Autodesk Inventor part; units mm, degrees
ref_plane "YZ Plane" through (0, 0, 0) normal (1, 0, 0) x (0, 1, 0)
ref_plane "XZ Plane" through (0, 0, 0) normal (0, 1, 0) x (-1, 0, 0)
ref_plane "XY Plane" through (0, 0, 0) normal (0, 0, 1) x (1, 0, 0)
sketch "スケッチ1" plane through (0, 0, 0) normal (0, 1, 0) x (-1, 0, 0)
  line L0 (0, 0) -> (15, 0)
  line L1 (40, 0) -> (40, -7.5) construction
  line L2 (40, -30) -> (15, -30) construction
  line L3 (0, -30) -> (0, 0)
  line L4 (40, -7.5) -> (40, -22.5)
  line L5 (40, -7.5) -> (55, -7.5) construction
  line L6 (40, -22.5) -> (15, -30)
  line L7 (40, -7.5) -> (15, 0)
  line L8 (15, 0) -> (40, 0) construction
  line L9 (40, -7.5) -> (40, -22.5)
  line L10 (40, -22.5) -> (40, -30) construction
  line L11 (15, -30) -> (0, -30)
  dimension "d0" = 40
  dimension "d1" = 30
  dimension "d2" = 7.5
  dimension "d3" = 15
  dimension "d4" = 90
  dimension "d5" = 15
  dimension "d6" = 15
extrude "押し出し1" add sketch "スケッチ1" along normal blind 3
sketch "スケッチ2" plane through (0, 3, 0) normal (0, 1, 0) x (1, 0, 0)
  line L0 (0, 0) -> (0, 30)
  line L1 (-15, 0) -> (0, 0)
  point P0 (-35, 15)
  point P1 (-35, 15)
  point P2 (-25, 15)
  point P3 (-7.5, 15)
  point P4 (-7.5, 5)
  point P5 (-7.5, 25)
  dimension "d9" = 35
  dimension "d10" = 15
  dimension "d11" = 10
  dimension "d12" = 7.5
  dimension "d13" = 15
  dimension "d14" = 10
  dimension "d15" = 10
hole "穴1" at (-35, 3, -15) at (-25, 3, -15) at (-7.5, 3, -15) at (-7.5, 3, -5) at (-7.5, 3, -25) direction (0, -1, 0) diameter 3.2 end through all
fillet "フィレット1" radius 2 6 edges at (-15, 1.5, 0) (0, 1.5, 0) (0, 1.5, -30) (-40, 1.5, -7.5) (-40, 1.5, -22.5) (-15, 1.5, -30)
properties part number "射出_固定5" material "アルミニウム 6061"
Part model, mm, in its own coordinate system. Round coordinates to 2 decimals unless told otherwise and drop trailing zeros. Order: outer loops, then holes, each group sorted by start corner. A loop starts at its lowest first (then second) coordinate and runs counter-clockwise, first axis right, second up. Notation, with made-up numbers: M 21,85.25 L 64,85.25 A23 ccw 64,121.25 Z; hole C 36,7.5 d1. An arc over 180 degrees is marked long. Answer in a Markdown table with one row per item. Add a question column.
Q1. Wall check: L1, parallel to X at y = 0.9, z = -15; L2, parallel to Z at x = -25, y = 1.9; L3, parallel to Z at x = -35, y = 1.1. Give the ranges that are in metal, low to high. Write a range as from..to.
Q2. Cut at B-B on y = 2.5. Give the cut face in (x, z).
Q3. Cut at D-D on z = -25. Give the cut face in (x, y).
Q4. Pin check, flat tips, straight feed: pin 1 (3.5 mm diameter, centred on x = -7.5, z = -5, fed in from -Y); pin 2 (2.5 mm diameter, centred on x = -7.5, z = -25, fed in from +Y); pin 3 (1.5 mm diameter, centred on x = -23, y = 1, fed in from -Z) (3 decimals); pin 4 (1 mm diameter, centred on x = -26, y = 0.5, fed in from +Z). Stop position of each tip, or through.
Q5. Cut at A-A on x = -7.5. Give the cut face in (y, z).
Q6. Mould opens along X. For faces 1 (the face through (-6.53, 1.48, -16.27)), 2 (the face through (-27.091, 1.479, -3.627)), 3 (the face through (-5.94, 1.48, -5.35)), 4 (the face through (-0.57, 1.52, -29.4)) say: +X half, -X half, draft (parallel to the pull), parting line (faces both ways), or undercut.
Q7. Cut at C-C on x = -36. Give the cut face in (y, z), and give its area (3 significant figures).
Established:
| question | item | result |
|---|---|---|
| 1 | L1 | x = -40..-36.6, -33.4..-26.6, -23.4..-9.1, -5.9..0 |
| 1 | L2 | z = -27..-16.6, -13.4..-3 |
| 1 | L3 | z = -24..-16.6, -13.4..-6 |
| 2 | outline | M -40,-21.01 A2 ccw -38.57,-22.93 L -15.28,-29.92 A2 ccw -14.71,-30 L -2,-30 A2 ccw 0,-28 L 0,-2 A2 ccw -2,0 L -14.71,0 A2 ccw -15.28,-0.08 L -38.57,-7.07 A2 ccw -40,-8.99 Z; hole C -35,-15 d3.2; hole C -25,-15 d3.2; hole C -7.5,-25 d3.2; hole C -7.5,-15 d3.2; hole C -7.5,-5 d3.2 |
| 3 | outline | M -31.67,0 L -9.1,0 L -9.1,3 L -31.67,3 Z; M -5.9,0 L 0,0 L 0,3 L -5.9,3 Z |
| 4 | pin 1 | stops at y = 0 |
| 4 | pin 2 | passes through |
| 4 | pin 3 | stops at z = -27.825 |
| 4 | pin 4 | stops at z = -3.15 |
| 5 | outline | M 0,-30 L 3,-30 L 3,-26.6 L 0,-26.6 Z; M 0,-23.4 L 3,-23.4 L 3,-16.6 L 0,-16.6 Z; M 0,-13.4 L 3,-13.4 L 3,-6.6 L 0,-6.6 Z; M 0,-3.4 L 3,-3.4 L 3,0 L 0,0 Z |
| 6 | face 1 | undercut |
| 6 | face 2 | -X half |
| 6 | face 3 | undercut |
| 6 | face 4 | +X half |
| 7 | outline | M 0,-23.7 L 3,-23.7 L 3,-16.25 L 0,-16.25 Z; M 0,-13.75 L 3,-13.75 L 3,-6.3 L 0,-6.3 Z |
| 7 | area | 44.7 mm2 |
